The listing builds one solid part. Answer for the finished solid, in the listing's coordinates (mm). Face numbers are marked on the shaded views. Give positions to 0.01 mm unless a question says otherwise; leave off trailing zeros. Order: outer loops, then holes, each group sorted by start corner. A loop starts at its lowest first (then second) coordinate and runs counter-clockwise, first axis right, second up. Notation, with made-up numbers: (31, -1.5) - (45, -1.5) arc R8 cw to (45, 3.5) - close; hole circle Ø9 at (60.5, 68). An arc over 180 degrees is marked (long way). Answer in a Markdown table with one row per item. Add a question column.
```python
from build123d import *

# Parameters (mm, degrees)
CROQUIS6_W              = 150
CROQUIS6_H              = 135
SALIENTE_EXTRUIR6_DEPTH = 2
CROQUIS8_W              = 5
CROQUIS8_H              = 10
CROQUIS8_W_2            = 10
CROQUIS8_R              = 1.5
SALIENTE_EXTRUIR7_DEPTH = 15
CROQUIS9_R              = 1.5
CORTAR_EXTRUIR1_DEPTH   = 10
CORTAR_EXTRUIR2_START   = -10
CROQUIS10_R             = 1.5
CORTAR_EXTRUIR2_DEPTH   = 10


with BuildPart() as part:
    # Croquis6 → Saliente-Extruir6 (new body)
    with BuildSketch(Plane(origin=(0, 0, 0), x_dir=(1, 0, 0), z_dir=(0, 1, 0))):
        with Locations((75, 67.5)):
            Rectangle(CROQUIS6_W, CROQUIS6_H)
    extrude(amount=-SALIENTE_EXTRUIR6_DEPTH)

    # Croquis8 → Saliente-Extruir7 (add)
    # profile 1 of 7: a face of its own
    with BuildSketch(Plane(origin=(0, 0, 0), x_dir=(1, 0, 0), z_dir=(0, 1, 0))):
        with Locations((4.5, 124)):
            Rectangle(CROQUIS8_W, CROQUIS8_H)
    # profile 2 of 7: a face of its own
    with BuildSketch(Plane(origin=(0, 0, 0), x_dir=(1, 0, 0), z_dir=(0, 1, 0))):
        with Locations((4.5, 7)):
            Rectangle(CROQUIS8_W, CROQUIS8_H)
    # profile 3 of 7: a face of its own
    with BuildSketch(Plane(origin=(0, 0, 0), x_dir=(1, 0, 0), z_dir=(0, 1, 0))):
        with Locations((143, 128)):
            Rectangle(CROQUIS8_W_2, CROQUIS8_H)
    # profile 4 of 7: a face of its own
    with BuildSketch(Plane(origin=(0, 0, 0), x_dir=(1, 0, 0), z_dir=(0, 1, 0))):
        with Locations((143, 7)):
            Rectangle(CROQUIS8_W_2, CROQUIS8_H)
    # profile 5 of 7: a face of its own
    with BuildSketch(Plane(origin=(0, 0, 0), x_dir=(1, 0, 0), z_dir=(0, 1, 0))):
        with Locations((139, 35)):
            Rectangle(CROQUIS8_W_2, CROQUIS8_H)
        with Locations(Location((139, 35, 0), (0, 0, 270))):
            Circle(CROQUIS8_R, mode=Mode.SUBTRACT)
    # profile 6 of 7: a face of its own
    with BuildSketch(Plane(origin=(0, 0, 0), x_dir=(1, 0, 0), z_dir=(0, 1, 0))):
        with Locations((17, 36)):
            Rectangle(CROQUIS8_W_2, CROQUIS8_H)
        with Locations(Location((17, 36, 0), (0, 0, 270))):
            Circle(CROQUIS8_R, mode=Mode.SUBTRACT)
    # profile 7 of 7: a face of its own
    with BuildSketch(Plane(origin=(0, 0, 0), x_dir=(1, 0, 0), z_dir=(0, 1, 0))):
        with Locations((99, 124)):
            Rectangle(CROQUIS8_W_2, CROQUIS8_H)
        with Locations(Location((99, 124, 0), (0, 0, 270))):
            Circle(CROQUIS8_R, mode=Mode.SUBTRACT)
    extrude(amount=SALIENTE_EXTRUIR7_DEPTH)

    # Croquis9 → Cortar-Extruir1 (cut)
    with BuildSketch(Plane.ZY):
        with Locations((-124, 10)):
            Circle(CROQUIS9_R)
        with Locations((-7, 10)):
            Circle(CROQUIS9_R)
    extrude(amount=-CORTAR_EXTRUIR1_DEPTH, mode=Mode.SUBTRACT)

    # Croquis10 → Cortar-Extruir2 (cut)
    with BuildSketch(Plane(origin=(148, 0, 0), x_dir=(0, 0, -1), z_dir=(1, 0, 0)).offset(CORTAR_EXTRUIR2_START)):
        with Locations(Location((7, 10, 0), (0, 0, 180))):
            Circle(CROQUIS10_R)
        with Locations((128, 10)):
            Circle(CROQUIS10_R)
    extrude(amount=CORTAR_EXTRUIR2_DEPTH, mode=Mode.SUBTRACT)


solid = part.part
```
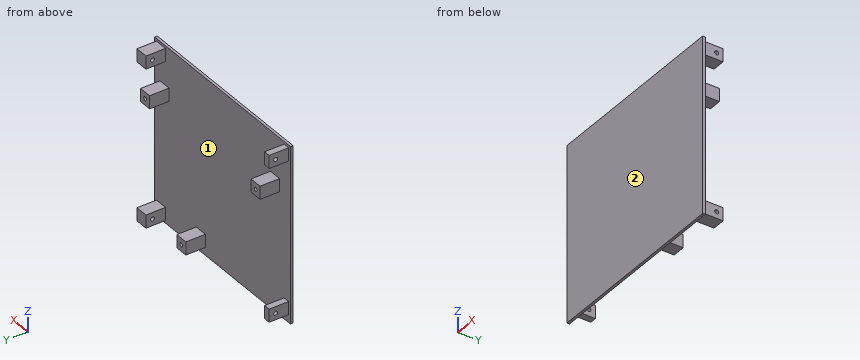
(1) Find section B-B, the plane z = -79. Write down the section's boundary in (x, y), plus the area to 3 significant figures.
(2) Each of these flat-tipped pins is pushed along its axis until it touches: P1, Ø3, axis at y = 10.5, z = -129.5, coming from the +X side; P2, Ø1.8, axis at y = 10, z = -7, coming from the +X side; P3, Ø8, axis at y = 8.5, z = -37, coming from the -X side; P4, Ø2.5, axis at y = 10, z = -124, coming from the -X side. Where does it stop, or does it pass through?
(3) The mould has two halves that part along X. Classify the marked faces 1 and 2: +X half, -X half, draft (parallel to the pull), parting line (faces both ways), or undercut.
(4) Straight lines are drawn through the part: line 1 (Y direction, x = 5.9, z = -7); line 2 (X direction, y = 8.5, z = -36); line 3 (Z direction, x = 99, y = 10.75). For each, find the intervals that lie inside material, in ascending order.
(5) Find section A-A, the plane y = 5.25. Give the number of separate pieces and of enclosed holes in the cut face, plus the area to 3 significant figures.
(6) Find section C-C, the plane x = 122. Write down the section's boundary in (y, z).
Answer key:
| question | item | result |
|---|---|---|
| 1 | outline | (0, -2) - (150, -2) - (150, 0) - (0, 0) - close |
| 1 | area | 300 mm² |
| 2 | P1 | x = 148 |
| 2 | P2 | through |
| 2 | P3 | x = 12 |
| 2 | P4 | x = 94 |
| 3 | face 1 | undercut |
| 3 | face 2 | draft |
| 4 | line 1 | -2 to 8.5, 11.5 to 15 |
| 4 | line 2 | 12 to 15.5, 18.5 to 22, 134 to 137.88, 140.12 to 144 |
| 4 | line 3 | -129 to -125.5, -122.5 to -119 |
| 5 | separate pieces | 7 |
| 5 | enclosed holes | 3 |
| 5 | area | 579 mm² |
| 6 | outline | (-2, -135) - (0, -135) - (0, 0) - (-2, 0) - close |
